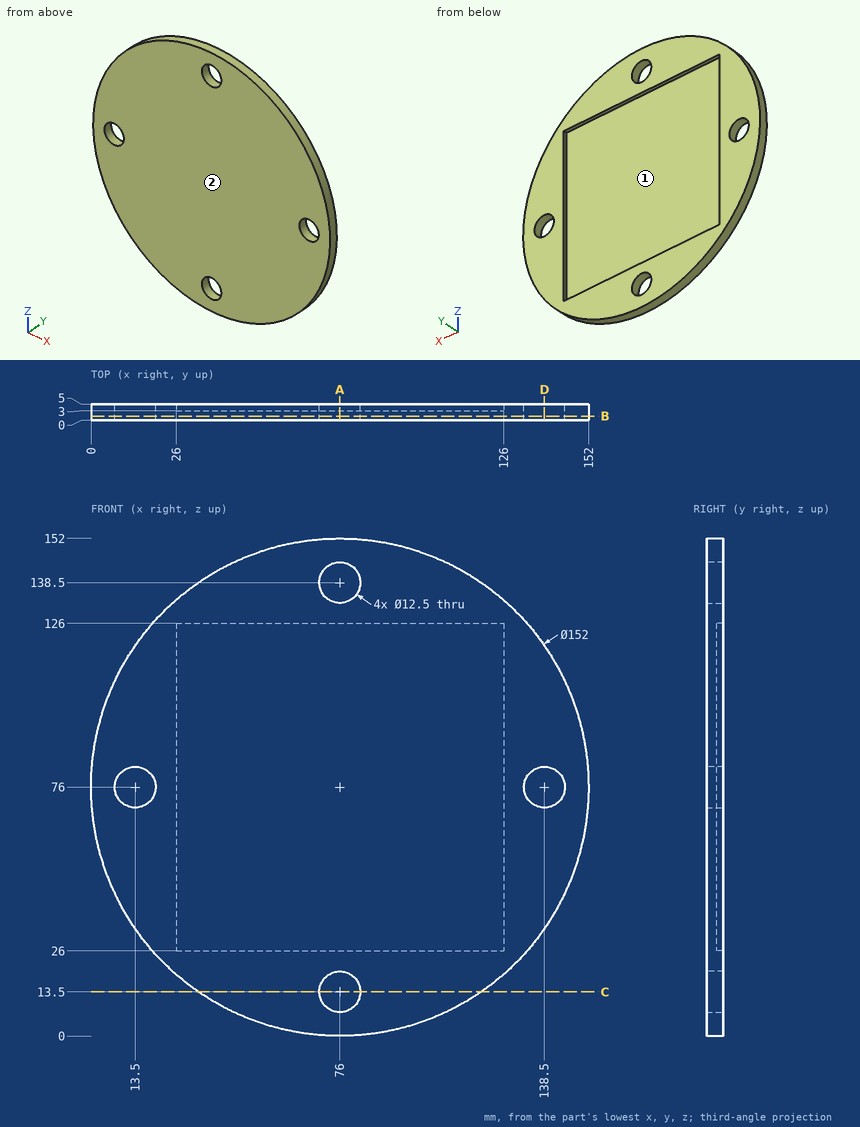
Job drawing, mm, ordinate dimensions from the low corner. One solid piece. Coordinates: 2 decimals unless noted, no trailing zeros. Loops run counter-clockwise (first coordinate to the right, second up) from the corner with the lowest first, then second, coordinate; pieces in that order, holes last. Notation, with made-up numbers: (-35.5, 10.5) - (-15.5, 10.5) arc R29 cw to (-15.5, 32.5) - close; hole circle Ø5 at (-8.75, 89.5). An arc over 180 degrees is marked (long way). Write item = value, one per line. Start each with the question number.
Q1. Drill centre lines: L1, parallel to X at y = 2.35, z = 76; L2, parallel to Y at x = 122, z = 29.5; L3, parallel to X at y = 1.25, z = 19. Where is each one in solid material? Low to high.
Q2. Cut at B-B, the plane y = 1.3. List the corners of the cut face in (x, z).
Q3. Flat gauge pins, fed straight in: pin 1 Ø2 at (x, y) = (95.5, 4.5) entering from -Z; pin 2 Ø7.5 at (x, z) = (13.5, 76) entering from -Y; pin 3 Ø0.6 at (y, z) = (3.5, 75) entering from -X; pin 4 Ø3 at (x, y) = (45, 2) entering from -Z. Where does each tip first touch, or does it go through?
Q4. Cut at C-C, the plane z = 13.5. List the corners of the cut face in (x, y).
Q5. Cut at D-D, the plane x = 138.5. List the corners of the cut face in (y, z), then the cut area to 3 significant figures.
Q6. Pull direction Z, two halves, no side cores. Call the marked faces 1 and 2: pulls with the +Z half, pulls with the -Z half, needs draft (parallel to the pull), parting line crosses it, or undercut.
Q7. Cut at A-A, the plane x = 76. List the corners of the cut face in (y, z).
Computed:
q1.L1 = 0 to 7.25, 19.75 to 132.25, 144.75 to 152
q1.L2 = 0 to 3
q1.L3 = 25.73 to 73.03, 78.97 to 126.27
q2.outline = circle Ø152 at (76, 76); hole circle Ø12.5 at (13.5, 76); hole circle Ø12.5 at (76, 13.5); hole circle Ø12.5 at (76, 138.5); hole circle Ø12.5 at (138.5, 76)
q3.pin_1 = 2.29
q3.pin_2 = through
q3.pin_3 = 0
q3.pin_4 = 5.96
q4.outline = (32.76, 0) - (69.75, 0) - (69.75, 5) - (32.76, 5) - close; (82.25, 0) - (119.24, 0) - (119.24, 5) - (82.25, 5) - close
q5.outline = (0, 32.76) - (5, 32.76) - (5, 69.75) - (0, 69.75) - close; (0, 82.25) - (5, 82.25) - (5, 119.24) - (0, 119.24) - close
q5.area = 370 mm²
q6.face_1 = undercut
q6.face_2 = needs draft
q7.outline = (0, 0) - (5, 0) - (5, 7.25) - (0, 7.25) - close; (0, 19.75) - (5, 19.75) - (5, 26) - (3, 26) - (3, 126) - (5, 126) - (5, 132.25) - (0, 132.25) - close; (0, 144.75) - (5, 144.75) - (5, 152) - (0, 152) - close
